from build123d import *

# Parameters (mm, degrees)
SKETCH3_R           = 3.15
BOSS_EXTRUDE1_DEPTH = 5
SKETCH4_R           = 2.5
BOSS_EXTRUDE2_DEPTH = 150
BOSS_EXTRUDE3_DEPTH = 5


with BuildPart() as part:
    # Sketch3 → Boss-Extrude1 (new body)
    with BuildSketch(Plane.XY):
        with BuildLine():
            ThreePointArc((9.448282799, 1.1), (7.983816705, 4.635533906), (4.448282799, 6.1))
            Line((4.448282799, 6.1), (-4.448282849, 6.1))
            ThreePointArc((-4.448282849, 6.1), (-7.983816755, 4.635533906), (-9.448282849, 1.1))
            Line((-9.448282849, 1.1), (-9.448282849, -8.15))
            Line((-9.448282849, -8.15), (9.448282799, -8.15))
            Line((9.448282799, -8.15), (9.448282799, 1.1))
        make_face()
        Circle(SKETCH3_R, mode=Mode.SUBTRACT)
    extrude(amount=BOSS_EXTRUDE1_DEPTH)

    # Sketch4 → Boss-Extrude2 (add)
    with BuildSketch(Plane(origin=(0, 6.1, 0), x_dir=(1, 0, 0), z_dir=(0, 1, 0))):
        with Locations(Location((0, -2.5, 0), (0, 0, 270))):
            Circle(SKETCH4_R)
    extrude(amount=BOSS_EXTRUDE2_DEPTH)

    # Sketch6 → Cut-Revolve2 (revolve, cut)
    with BuildSketch(Plane(origin=(0, 0, 0), x_dir=(0, 0, -1), z_dir=(1, 0, 0))):
        Polygon((-2.5, 157.475466352), (-2.5, 156.1), (0, 150.602856099), (2.064701239, 157.475466352), align=None)
    revolve(axis=Axis((0, 156.1, 2.5), (0, 1, 0)), mode=Mode.SUBTRACT)

    # Sketch7 → Boss-Extrude3 (add)
    with BuildSketch(Plane(origin=(0, 0, 0), x_dir=(-1, 0, 0), z_dir=(0, 0, -1))):
        Polygon((0, 26.076539937), (4.448282849, 6.1), (-4.448282799, 6.1), align=None)
    extrude(amount=-BOSS_EXTRUDE3_DEPTH)


solid = part.part
Build history of the part. All positions in model axes, mm. Coordinates: 2 decimals unless noted, no trailing zeros. Order: outer loops, then holes, each group sorted by start corner. A loop starts at its lowest first (then second) coordinate and runs counter-clockwise, first axis right, second up. Notation, with made-up numbers: (87.5, -7) - (109.5, -7) arc R8 cw to (109.5, 3) - close; hole circle Ø5 at (37, 7.25). An arc over 180 degrees is marked (long way). Put each result on its own line as item: value.
1. Probe line 1 along Z through (x, y) = (-0.25, 127); line 2 along X through (y, z) = (94, 2.1); line 3 along Y through (x, z) = (0, 1.85). List the from-to ranges inside material, lowest first. Write a range as [from, to].
Answer sheet:
line 1: z = [0.01, 4.99]
line 2: x = [-2.47, 2.47]
line 3: y = [-8.15, -3.15], [3.15, 154.67]
2. Drop flat-ended pins along their axis: P1, Ø6, axis at x = 3, y = 99, coming from the +Z side; P2, Ø3, axis at x = 1.5, z = 3.5, coming from the +Y side. Give the stop position or say it passes through.
Answer sheet:
P1: stops at z = 5
P2: stops at y = 155.43
3. Saw through at B-B (y = 23). Write the cut outline in (x, z), and give its area (3 significant figures).
Answer sheet:
outline: (-0.69, 0) - (0.69, 0) - (0.69, 0.1) arc R2.5 ccw to (0.69, 4.9) - (0.69, 5) - (-0.69, 5) - (-0.69, 4.9) arc R2.5 ccw to (-0.69, 0.1) - close
area: 19.7 mm^2
4. Saw through at A-A (y = 101). Write the cut outline in (x, z), and give its area (3 significant figures).
Answer sheet:
outline: circle Ø5 at (0, 2.5)
area: 19.6 mm^2
5. Pull direction Y, two halves, no side cores. Call faces 1 (the face through (0, 82, 0)), 2 (the face through (-7.945, 4.674, 2.465)), 3 (the face through (-2.5, -1.917, 2.465)): pulls with the +Y half, pulls with the -Y half, needs draft (parallel to the pull), parting line crosses it, or undercut.
Answer sheet:
face 1: needs draft
face 2: pulls with the +Y half
face 3: undercut
